Here's how the part is built. I have some questions about the finished solid (model axes, mm). Coordinates: 2 decimals unless noted, no trailing zeros. Write each loop counter-clockwise with the first axis right and the second up, starting at its lowest first coordinate (ties: lowest second). Pieces come first, ordered by that corner, then holes. Notation, with made-up numbers: (40, 71) -> (54, 71) arc R34 cw to (54, 108) -> close; hole circle Ø4 at (75.25, -12). An arc over 180 degrees is marked (long way). Use a Markdown table: item, result. Add a question column.
Item 1: Imagine slicing it at C-C, the plane x = -59. Write out the boundary of the cut face in (y, z), and give its area (3 significant figures).
Item 2: Imagine slicing it at B-B, the plane y = 2. Write out the boundary of the cut face in (x, z), and give its area (3 significant figures).
Item 3: Will these pins go through, and if not, where does the flat tip stop? pin 1 Ø0.9 at (x, y) = (57, 1.5) entering from -Z; pin 2 Ø1.5 at (y, z) = (2.5, -51) entering from +X; pin 3 Ø10 at (x, z) = (-29.5, -16.5) entering from -Y; pin 4 Ø0.9 at (x, y) = (57, 1.5) entering from +Z.
Item 4: Imagine slicing it at D-D, the plane z = 50. Write out the boundary of the cut face in (x, y).
Item 5: Imagine slicing it at A-A, the plane z = 0. Write out the boundary of the cut face in (x, y).
Item 6: If I drill on line 1 along X through (y, z) = (0.2, 12); line 2 along Z through (x, y) = (0, 0.6); line 3 along Z through (x, y) = (58, 2.3), over which ranges is the centre line in solid material (lowest first)? Write a range as from..to.
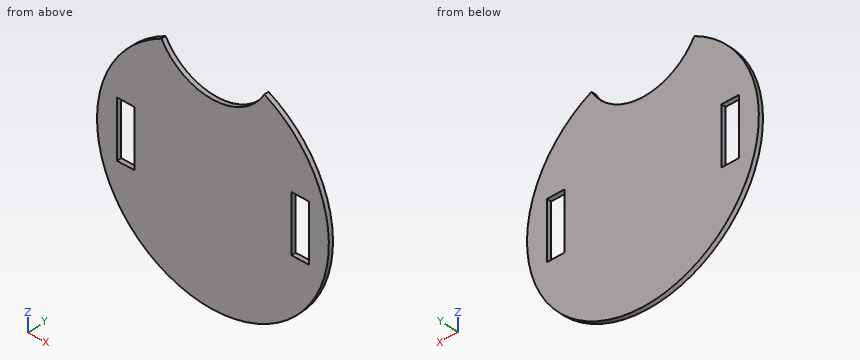
```python
from build123d import *

# Parameters (mm, degrees)
BOSS_EXTRUDE1_DEPTH = 2.9
SKETCH2_W           = 11.27569817
SKETCH2_H           = 36.991766838
CUT_EXTRUDE1_DEPTH  = 107.105654892


with BuildPart() as part:
    # Sketch1 → Boss-Extrude1 (new body)
    with BuildSketch(Plane(origin=(0, 0, 0), x_dir=(1, 0, 0), z_dir=(0, 1, 0))):
        with BuildLine():
            ThreePointArc((33.29110537, -67.206415641), (0, 75), (-33.29110537, -67.206415641))
            ThreePointArc((-33.29110537, -67.206415641), (0, -47.791616815), (33.29110537, -67.206415641))
        make_face()
    extrude(amount=BOSS_EXTRUDE1_DEPTH)

    # Sketch2 → Cut-Extrude1 (cut, through all)
    with BuildSketch(Plane(origin=(0, 2.9, 0), x_dir=(1, 0, 0), z_dir=(0, 1, 0))):
        with Locations((-56.433097695, -0.165843751)):
            Rectangle(SKETCH2_W, SKETCH2_H)
        with Locations((56.433097695, -0.165843751)):
            Rectangle(SKETCH2_W, SKETCH2_H)
    extrude(amount=-CUT_EXTRUDE1_DEPTH, mode=Mode.SUBTRACT)


solid = part.part
```
Ans:
| question | item | result |
|---|---|---|
| 1 | outline | (0, -46.3) -> (2.9, -46.3) -> (2.9, -18.33) -> (0, -18.33) -> close; (0, 18.66) -> (2.9, 18.66) -> (2.9, 46.3) -> (0, 46.3) -> close |
| 1 | area | 161 mm^2 |
| 2 | outline | (-33.29, 67.21) arc R75 ccw (long way) to (33.29, 67.21) arc R38.25 cw to start; hole (-62.07, -18.33) -> (-50.8, -18.33) -> (-50.8, 18.66) -> (-62.07, 18.66) -> close; hole (50.8, -18.33) -> (62.07, -18.33) -> (62.07, 18.66) -> (50.8, 18.66) -> close |
| 2 | area | 15,600 mm^2 |
| 3 | pin 1 | stops at z = -49.27 |
| 3 | pin 2 | stops at x = 55.68 |
| 3 | pin 3 | stops at y = 0 |
| 3 | pin 4 | stops at z = 49.27 |
| 4 | outline | (-55.9, 0) -> (-12.81, 0) -> (-12.81, 2.9) -> (-55.9, 2.9) -> close; (12.81, 0) -> (55.9, 0) -> (55.9, 2.9) -> (12.81, 2.9) -> close |
| 5 | outline | (-75, 0) -> (-62.07, 0) -> (-62.07, 2.9) -> (-75, 2.9) -> close; (-50.8, 0) -> (50.8, 0) -> (50.8, 2.9) -> (-50.8, 2.9) -> close; (62.07, 0) -> (75, 0) -> (75, 2.9) -> (62.07, 2.9) -> close |
| 6 | line 1 | x = -74.03..-62.07, -50.8..50.8, 62.07..74.03 |
| 6 | line 2 | z = -75..47.79 |
| 6 | line 3 | z = -47.55..-18.33, 18.66..47.55 |
